Verification items for this drawing (mm, ordinates from the low corner). Round coordinates to 2 decimals unless told otherwise and drop trailing zeros. Order: outer loops, then holes, each group sorted by start corner. A loop starts at its lowest first (then second) coordinate and runs counter-clockwise, first axis right, second up. Notation, with made-up numbers: (57, 43) -> (74, 43) arc R16 cw to (74, 54) -> close; hole circle Ø5 at (15, 70). An arc over 180 degrees is marked (long way). Return JSON: item names as keys, results as strings. Group by question number.
Item 1: Sectioned sample at A-A on x = 97. Record the cut outline in (y, z), plus the area to 3 significant figures.
Item 2: Depth check by flat-ended pin: pin 1 Ø1.5 at (y, z) = (41, 2.5) entering from -X; pin 2 Ø10 at (y, z) = (54, 183) entering from -X; pin 3 Ø5 at (y, z) = (37.5, 219.5) entering from +X. Enter the tip coordinate at first touch or a pass-through.
Item 3: Sectioned sample at B-B on y = 54.5. Record the cut outline in (x, z), plus the area to 3 significant figures.
Item 4: Sectioned sample at C-C on z = 49. Record the cut outline in (x, y).
Item 5: Scan lines: probe 1 along X at (y, z) = (63, 41); probe 2 along Z at (x, y) = (41.5, 76). Record each from-to range of solid material in increasing order. Write a range as from..to.
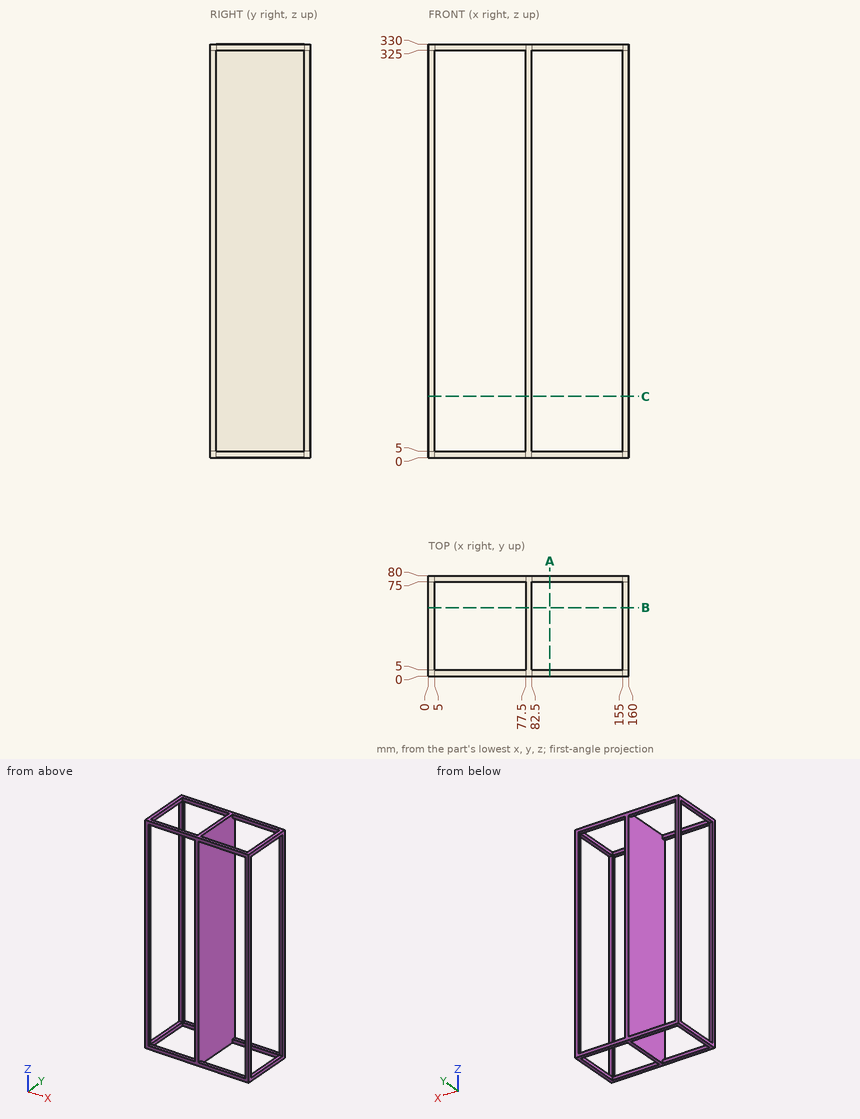
Recorded:
{
 "1": {"outline": "(0, 0) -> (5, 0) -> (5, 5) -> (0, 5) -> close; (0, 325) -> (5, 325) -> (5, 330) -> (0, 330) -> close; (75, 0) -> (80, 0) -> (80, 5) -> (75, 5) -> close; (75, 325) -> (80, 325) -> (80, 330) -> (75, 330) -> close", "area": "100 mm²"},
 "2": {"pin 1": "x = 0", "pin 2": "x = 77.5", "pin 3": "x = 82.5"},
 "3": {"outline": "(0, 0) -> (5, 0) -> (5, 5) -> (0, 5) -> close; (0, 325) -> (5, 325) -> (5, 330) -> (0, 330) -> close; (77.5, 0) -> (82.5, 0) -> (82.5, 330) -> (77.5, 330) -> close; (155, 0) -> (160, 0) -> (160, 5) -> (155, 5) -> close; (155, 325) -> (160, 325) -> (160, 330) -> (155, 330) -> close", "area": "1,750 mm²"},
 "4": {"outline": "(0, 0) -> (5, 0) -> (5, 5) -> (0, 5) -> close; (0, 75) -> (5, 75) -> (5, 80) -> (0, 80) -> close; (77.5, 0) -> (82.5, 0) -> (82.5, 80) -> (77.5, 80) -> close; (155, 0) -> (160, 0) -> (160, 5) -> (155, 5) -> close; (155, 75) -> (160, 75) -> (160, 80) -> (155, 80) -> close"},
 "5": {"probe 1": "77.5..82.5", "probe 2": "0..5, 325..330"}
}
